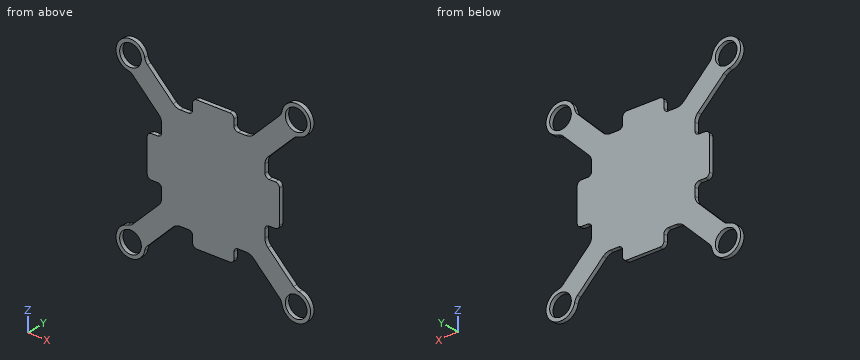
from build123d import *

# Parameters (mm, degrees)
SKETCH_1_R      = 5.25
EXTRUDE_1_DEPTH = 2


with BuildPart() as part:
    # 草图1 → 凸台-拉伸1 (new body)
    with BuildSketch(Plane(origin=(0, 0, 0), x_dir=(1, 0, 0), z_dir=(0, 1, 0))):
        with BuildLine():
            Line((-15.928932188, -25), (-12, -25))
            ThreePointArc((-12, -25), (-10.585786438, -25.585786438), (-10, -27))
            Line((-10, -27), (-10, -30))
            ThreePointArc((-10, -30), (-9.414213562, -31.414213562), (-8, -32))
            Line((-8, -32), (8, -32))
            ThreePointArc((8, -32), (9.414213562, -31.414213562), (10, -30))
            Line((10, -30), (10, -27))
            ThreePointArc((10, -27), (10.585786438, -25.585786438), (12, -25))
            Line((12, -25), (15.928932188, -25))
            ThreePointArc((15.928932188, -25), (17.84234935, -25.380602337), (19.464466094, -26.464466094))
            Line((19.464466094, -26.464466094), (31.856955479, -38.856955479))
            ThreePointArc((31.856955479, -38.856955479), (32.735932701, -40.044705003), (33.229373027, -41.437495918))
            ThreePointArc((33.229373027, -41.437495918), (45.050252532, -45.050252532), (41.437495918, -33.229373027))
            ThreePointArc((41.437495918, -33.229373027), (40.044705003, -32.735932701), (38.856955479, -31.856955479))
            Line((38.856955479, -31.856955479), (26.464466094, -19.464466094))
            ThreePointArc((26.464466094, -19.464466094), (25.380602337, -17.84234935), (25, -15.928932188))
            Line((25, -15.928932188), (25, -12))
            ThreePointArc((25, -12), (25.585786438, -10.585786438), (27, -10))
            Line((27, -10), (30, -10))
            ThreePointArc((30, -10), (31.414213562, -9.414213562), (32, -8))
            Line((32, -8), (32, 8))
            ThreePointArc((32, 8), (31.414213562, 9.414213562), (30, 10))
            Line((30, 10), (27, 10))
            ThreePointArc((27, 10), (25.585786438, 10.585786438), (25, 12))
            Line((25, 12), (25, 15.928932188))
            ThreePointArc((25, 15.928932188), (25.380602337, 17.84234935), (26.464466094, 19.464466094))
            Line((26.464466094, 19.464466094), (38.856955479, 31.856955479))
            ThreePointArc((38.856955479, 31.856955479), (40.044705003, 32.735932701), (41.437495918, 33.229373027))
            ThreePointArc((41.437495918, 33.229373027), (45.050252532, 45.050252532), (33.229373027, 41.437495918))
            ThreePointArc((33.229373027, 41.437495918), (32.735932701, 40.044705003), (31.856955479, 38.856955479))
            Line((31.856955479, 38.856955479), (19.464466094, 26.464466094))
            ThreePointArc((19.464466094, 26.464466094), (17.84234935, 25.380602337), (15.928932188, 25))
            Line((15.928932188, 25), (12, 25))
            ThreePointArc((12, 25), (10.585786438, 25.585786438), (10, 27))
            Line((10, 27), (10, 30))
            ThreePointArc((10, 30), (9.414213562, 31.414213562), (8, 32))
            Line((8, 32), (-8, 32))
            ThreePointArc((-8, 32), (-9.414213562, 31.414213562), (-10, 30))
            Line((-10, 30), (-10, 27))
            ThreePointArc((-10, 27), (-10.585786438, 25.585786438), (-12, 25))
            Line((-12, 25), (-15.928932188, 25))
            ThreePointArc((-15.928932188, 25), (-17.84234935, 25.380602337), (-19.464466094, 26.464466094))
            Line((-19.464466094, 26.464466094), (-31.856955479, 38.856955479))
            ThreePointArc((-31.856955479, 38.856955479), (-32.735932701, 40.044705003), (-33.229373027, 41.437495918))
            ThreePointArc((-33.229373027, 41.437495918), (-45.050252532, 45.050252532), (-41.437495918, 33.229373027))
            ThreePointArc((-41.437495918, 33.229373027), (-40.044705003, 32.735932701), (-38.856955479, 31.856955479))
            Line((-38.856955479, 31.856955479), (-26.464466094, 19.464466094))
            ThreePointArc((-26.464466094, 19.464466094), (-25.380602337, 17.84234935), (-25, 15.928932188))
            Line((-25, 15.928932188), (-25, 12))
            ThreePointArc((-25, 12), (-25.585786438, 10.585786438), (-27, 10))
            Line((-27, 10), (-30, 10))
            ThreePointArc((-30, 10), (-31.414213562, 9.414213562), (-32, 8))
            Line((-32, 8), (-32, -8))
            ThreePointArc((-32, -8), (-31.414213562, -9.414213562), (-30, -10))
            Line((-30, -10), (-27, -10))
            ThreePointArc((-27, -10), (-25.585786438, -10.585786438), (-25, -12))
            Line((-25, -12), (-25, -15.928932188))
            ThreePointArc((-25, -15.928932188), (-25.380602337, -17.84234935), (-26.464466094, -19.464466094))
            Line((-26.464466094, -19.464466094), (-38.856955479, -31.856955479))
            ThreePointArc((-38.856955479, -31.856955479), (-40.044705003, -32.735932701), (-41.437495918, -33.229373027))
            ThreePointArc((-41.437495918, -33.229373027), (-45.050252532, -45.050252532), (-33.229373027, -41.437495918))
            ThreePointArc((-33.229373027, -41.437495918), (-32.735932701, -40.044705003), (-31.856955479, -38.856955479))
            Line((-31.856955479, -38.856955479), (-19.464466094, -26.464466094))
            ThreePointArc((-19.464466094, -26.464466094), (-17.84234935, -25.380602337), (-15.928932188, -25))
        make_face()
        with Locations(Location((-40.100505063, 40.100505063, 0), (0, 0, 270))):
            Circle(SKETCH_1_R, mode=Mode.SUBTRACT)
        with Locations(Location((40.100505063, 40.100505063, 0), (0, 0, 270))):
            Circle(SKETCH_1_R, mode=Mode.SUBTRACT)
        with Locations(Location((40.100505063, -40.100505063, 0), (0, 0, 270))):
            Circle(SKETCH_1_R, mode=Mode.SUBTRACT)
        with Locations(Location((-40.100505063, -40.100505063, 0), (0, 0, 270))):
            Circle(SKETCH_1_R, mode=Mode.SUBTRACT)
    extrude(amount=EXTRUDE_1_DEPTH)


solid = part.part
CAD build for the part. Positions are in the model's coordinates, mm. Give positions to 0.01 mm unless a question says otherwise; leave off trailing zeros. Order: outer loops, then holes, each group sorted by start corner. A loop starts at its lowest first (then second) coordinate and runs counter-clockwise, first axis right, second up. Notation, with made-up numbers: (-1.5, -18) - (14.5, -18) arc R14 cw to (14.5, -6) - close; hole circle Ø1 at (87.25, -5.75). An arc over 180 degrees is marked (long way). Write each question's results on one line, items separated by ' | '.
1. Saw through at B-B on z = 37. List the corners of the cut face in (x, y), and give its area (3 significant figures).
Calculated:
outline: (-46.38, 0) - (-44.34, 0) - (-44.34, 2) - (-46.38, 2) - close; (-35.86, 0) - (-30, 0) - (-30, 2) - (-35.86, 2) - close; (30, 0) - (35.86, 0) - (35.86, 2) - (30, 2) - close; (44.34, 0) - (46.38, 0) - (46.38, 2) - (44.34, 2) - close | area: 31.6 mm2
2. Pin check, flat tips, straight feed: pin 1 (8.5 mm diameter, centred on x = -40.1, z = -40.1, fed in from -Y); pin 2 (1 mm diameter, centred on x = -2, y = 1, fed in from +Z); pin 3 (1 mm diameter, centred on y = 1, z = 13.5, fed in from -X); pin 4 (1 mm diameter, centred on y = 0.5, z = -0.5, fed in from +X). Stop position of each tip, or through.
Calculated:
pin 1: passes through | pin 2: stops at z = 32 | pin 3: stops at x = -25 | pin 4: stops at x = 32
3. Saw through at A-A on z = -28.5. List the corners of the cut face in (x, y), and give its area (3 significant figures).
Calculated:
outline: (-35.5, 0) - (-21.5, 0) - (-21.5, 2) - (-35.5, 2) - close; (-10, 0) - (10, 0) - (10, 2) - (-10, 2) - close; (21.5, 0) - (35.5, 0) - (35.5, 2) - (21.5, 2) - close | area: 96.0 mm2
4. Saw through at D-D on x = -23.5. List the corners of the cut face in (y, z), and give its area (3 significant figures).
Calculated:
outline: (0, -30.5) - (2, -30.5) - (2, 30.5) - (0, 30.5) - close | area: 122 mm2
5. Saw through at C-C on x = 37.5. List the corners of the cut face in (y, z), and give its area (3 significant figures).
Calculated:
outline: (0, -46.6) - (2, -46.6) - (2, -44.66) - (0, -44.66) - close; (0, -35.54) - (2, -35.54) - (2, -30.5) - (0, -30.5) - close; (0, 30.5) - (2, 30.5) - (2, 35.54) - (0, 35.54) - close; (0, 44.66) - (2, 44.66) - (2, 46.6) - (0, 46.6) - close | area: 27.9 mm2
6. Probe L1, parallel to X at y = 1.6, z = 28; L2, parallel to Z at x = 27, y = 0.15; L3, parallel to X at y = 0.4, z = 26. List the from-to ranges inside material, lowest first. Write a range as from..to.
Calculated:
L1: x = -35..-21, -10..10, 21..35 | L2: z = -34..-20, -10..10, 20..34 | L3: x = -33..-18.93, -10.27..10.27, 18.93..33
